Can you work these out from the model? Positions are in its coordinate system, mm. Face numbers are marked on the shaded views. Give positions to 0.01 mm unless a question says otherwise; leave off trailing zeros. Loops run counter-clockwise (first coordinate to the right, second up) from the corner with the lowest first, then second, coordinate; pieces in that order, holes last. Notation, with made-up numbers: (-25.5, 31) -> (11.5, 31) arc R23 cw to (11.5, 41) -> close; hole circle Ø2 at (67, 1). An arc over 180 degrees is marked (long way). One line per question, with ' | ' between items.
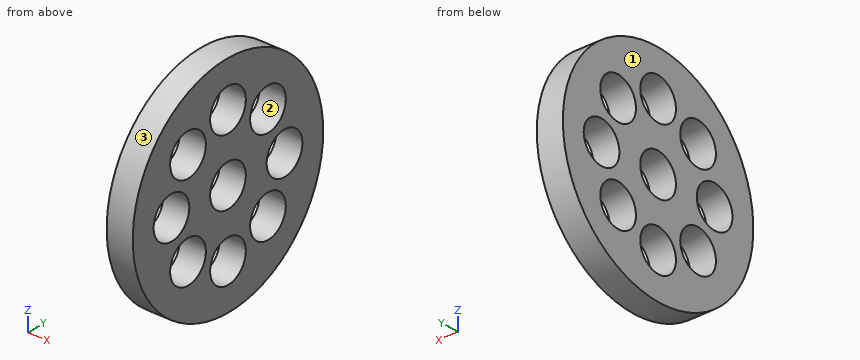
Autodesk Inventor part; units mm, degrees
ref_plane "YZ Plane" through (0, 0, 0) normal (1, 0, 0) x (0, 1, 0)
ref_plane "XZ Plane" through (0, 0, 0) normal (0, 1, 0) x (-1, 0, 0)
ref_plane "XY Plane" through (0, 0, 0) normal (0, 0, 1) x (1, 0, 0)
sketch "Sketch2" plane through (0, 0, 0) normal (1, 0, 0) x (0, 1, 0)
  circle A0 centre (0, 0) radius 20
  circle A1 centre (0, 0) radius 3.75
  circle A2 centre (11.875, 0) radius 3.75
  line L0 (20, 0) -> (15.625, 0) construction
  line L1 (8.125, 0) -> (3.75, 0) construction
  line L2 (0, 0) -> (3.75, 0) construction
  circle A3 centre (0, 11.875) radius 3.75
  circle A4 centre (-11.875, 0) radius 3.75
  circle A5 centre (0, -11.875) radius 3.75
  circle A6 centre (8.3969, 8.3969) radius 3.75
  circle A7 centre (0, 11.875) radius 3.75
  circle A8 centre (-8.3969, 8.3969) radius 3.75
  circle A9 centre (-11.875, 0) radius 3.75
  circle A10 centre (-8.3969, -8.3969) radius 3.75
  circle A11 centre (0, -11.875) radius 3.75
  circle A12 centre (8.3969, -8.3969) radius 3.75
  point P0 (0, 15.625)
  point P1 (0, 8.125)
  point P2 (-15.625, 0)
  point P3 (-8.125, 0)
  point P4 (0, -15.625)
  point P5 (0, -8.125)
  point P6 (11.0485, 11.0485)
  point P7 (5.7452, 5.7452)
  point P8 (0, 15.625)
  point P9 (0, 8.125)
  point P10 (-11.0485, 11.0485)
  point P11 (-5.7452, 5.7452)
  point P12 (-15.625, 0)
  point P13 (-8.125, 0)
  point P14 (-11.0485, -11.0485)
  point P15 (-5.7452, -5.7452)
  point P16 (0, -15.625)
  point P17 (0, -8.125)
  point P18 (11.0485, -11.0485)
  point P19 (5.7452, -5.7452)
  dimension "d0" = 40
  dimension "d1" = 7.5
  dimension "d6" = 360
  dimension "d10" = 360
  dimension "d12" = 7.5
extrude "Extrusion1" add sketch "Sketch2" along normal blind 4.7
properties part number "small_wheel_3DPrint"
Q1. If we mould it in two halves opening along Y, with no side actions, what happens to the marked faces 1, 2 and 3? For each: pulls with the +Y half, pulls with the -Y half, needs draft (parallel to the pull), parting line crosses it, or undercut.
Entries:
face 1: needs draft | face 2: undercut | face 3: parting line crosses it
Q2. If I drill on probe 1 along Z at (x, y) = (2.8, 0) (3 decimals); probe 2 along Y at (x, z) = (0.5, 8); probe 3 along Z at (x, y) = (3.5, -7.5), over which ranges is the centre line in solid material (lowest first)? Write a range as from..to.
Entries:
probe 1: -20..-15.625, -8.125..-3.75, 3.75..8.125, 15.625..20 | probe 2: -18.33..-12.13, -4.67..4.67, 12.13..18.33 | probe 3: -18.54..-12.04, -4.76..4.76, 12.04..18.54
Q3. For pin 1 Ø7 at (y, z) = (0, -11.875) entering from -X; pin 2 Ø1 at (x, y) = (4, -3.5) entering from -Z; pin 3 Ø2 at (x, y) = (1, -11) entering from +Z; pin 4 Ø1.5 at (x, z) = (2, 1) entering from +Y, each with a flat end and sliding along its axis, tell me the tip position at first contact or that it passes through.
Entries:
pin 1: through | pin 2: z = -19.77 | pin 3: z = 17.32 | pin 4: y = 20
Q4. If we section it at A-A (y = 0): Write out the boundary of the cut face in (x, z) (3 decimals), plus the area to 4 significant figures.
Entries:
outline: (0, -20) -> (4.7, -20) -> (4.7, -15.625) -> (0, -15.625) -> close; (0, -8.125) -> (4.7, -8.125) -> (4.7, -3.75) -> (0, -3.75) -> close; (0, 3.75) -> (4.7, 3.75) -> (4.7, 8.125) -> (0, 8.125) -> close; (0, 15.625) -> (4.7, 15.625) -> (4.7, 20) -> (0, 20) -> close | area: 82.25 mm²
Q5. If we section it at C-C (x = 0.6): State how many separate pieces and enclosed holes the cut face has, plus the area to 3 significant figures.
Entries:
separate pieces: 1 | enclosed holes: 9 | area: 859 mm²
Q6. If we section it at D-D (z = -14.5): Write out the boundary of the cut face in (x, y).
Entries:
outline: (0, -13.77) -> (4.7, -13.77) -> (4.7, -2.68) -> (0, -2.68) -> close; (0, 2.68) -> (4.7, 2.68) -> (4.7, 13.77) -> (0, 13.77) -> close
